Work out the finished part from the listing and answer in its coordinate system (mm). Face numbers are marked on the shaded views. A direction names the side the tool comes from. Coordinates: 2 decimals unless noted, no trailing zeros. Write each question's results on one line, items separated by ' | '. Start each with the question number.
Item 1: Section C-C, the plane y = 28.5 is taken. Count the separate pieces of the cut face and the enclosed holes in it, plus the area to 3 significant figures.
Item 2: Each of these flat-tipped pins is pushed along its axis until it touches: pin 1 Ø2.5 at (x, y) = (-1, 43.5) entering from +Z; pin 2 Ø3.5 at (x, z) = (65.5, -3.5) entering from -Y; pin 3 Ø13.5 at (x, y) = (-17, 24) entering from -Z. Where does it stop, or does it pass through?
Item 3: Consider probe 1 along Z at (x, y) = (-5.5, 29); probe 2 along Z at (x, y) = (-44, 42); probe 3 along X at (y, z) = (14, -38) (3 decimals). Determine where each line is inside the solid, lowest interval first. Write a range as [from, to].
Item 4: A tool of negligible diameter and unlimited length cuts with its end or side. For the marked faces 4, 5 and 6, from which of +Z, -Z, +X, -X, +Y, -Y can it reach the whole face along a straight path? Write none if from no direction.
Item 5: For a pull along Z with two mould halves and no side action, classify the marked faces 1, 2 and 3 as +Z half, -Z half, draft (parallel to the pull), parting line (faces both ways), or undercut.
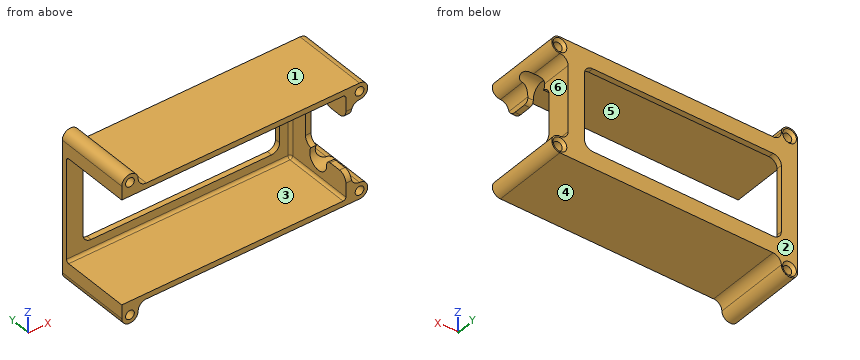
from build123d import *

# Parameters (mm, degrees)
SKETCH1_W           = 133.35
SKETCH1_H           = 66.675
SKETCH1_W_2         = 127
SKETCH1_H_2         = 60.325
BOSS_EXTRUDE1_DEPTH = 41.275
SKETCH2_W           = 31.75
SKETCH2_H           = 60.325
CUT_EXTRUDE1_DEPTH  = 134.35
SKETCH3_W           = 133.35
SKETCH3_H           = 66.675
SKETCH3_W_2         = 114.3
SKETCH3_H_2         = 47.625
BOSS_EXTRUDE2_DEPTH = 3.175
BOSS_EXTRUDE3_DEPTH = 44.45
SKETCH6_R           = 2.54
BOSS_EXTRUDE4_DEPTH = 44.45
CUT_EXTRUDE2_DEPTH  = 4.175
FILLET1_R           = 1.5875
FILLET2_R           = 4.7625
SKETCH9_R           = 6.35
CUT_EXTRUDE4_DEPTH  = 13.7
FILLET3_R           = 2.54


with BuildPart() as part:
    # Sketch1 → Boss-Extrude1 (new body)
    with BuildSketch(Plane(origin=(0, 0, 0), x_dir=(1, 0, 0), z_dir=(0, 1, 0))):
        Rectangle(SKETCH1_W, SKETCH1_H)
        Rectangle(SKETCH1_W_2, SKETCH1_H_2, mode=Mode.SUBTRACT)
    extrude(amount=BOSS_EXTRUDE1_DEPTH)

    # Sketch2 → Cut-Extrude1 (cut, through all)
    with BuildSketch(Plane.ZY.offset(66.675)):
        Rectangle(SKETCH2_W, SKETCH2_H)
    extrude(amount=-CUT_EXTRUDE1_DEPTH, mode=Mode.SUBTRACT)

    # Sketch3 → Boss-Extrude2 (add)
    with BuildSketch(Plane(origin=(0, 41.275, 0), x_dir=(1, 0, 0), z_dir=(0, 1, 0))):
        Rectangle(SKETCH3_W, SKETCH3_H)
        Rectangle(SKETCH3_W_2, SKETCH3_H_2, mode=Mode.SUBTRACT)
    extrude(amount=BOSS_EXTRUDE2_DEPTH)

    # Sketch4 → Boss-Extrude3 (add)
    with BuildSketch(Plane(origin=(0, 44.45, 0), x_dir=(1, 0, 0), z_dir=(0, 1, 0))):
        with BuildLine():
            Line((71.4375, 33.3375), (66.675, 33.3375))
            Line((66.675, 33.3375), (66.675, 19.05))
            ThreePointArc((66.675, 19.05), (68.069903955, 22.417596045), (71.4375, 23.8125))
            ThreePointArc((71.4375, 23.8125), (76.2, 28.575), (71.4375, 33.3375))
        make_face()
    boss_extrude3 = extrude(amount=-BOSS_EXTRUDE3_DEPTH)

    # Sketch5 → Cut-Revolve1 (revolve, cut)
    with BuildSketch(Plane.YZ.offset(71.4375)):
        Polygon((0, -31.115), (42.8625, -31.115), (44.45, -32.569675739), (44.45, -28.575), (0, -28.575), align=None)
    cut_revolve1 = revolve(axis=Axis((71.4375, 44.45, -28.575), (0, -1, 0)), mode=Mode.SUBTRACT)

    # Sketch6 → Boss-Extrude4 (add)
    with BuildSketch(Plane(origin=(0, 44.45, 0), x_dir=(1, 0, 0), z_dir=(0, 1, 0))):
        with BuildLine():
            Line((-66.675, 38.1), (-66.675, 33.3375))
            Line((-66.675, 33.3375), (-52.3875, 33.3375))
            ThreePointArc((-52.3875, 33.3375), (-55.755096045, 34.732403955), (-57.15, 38.1))
            ThreePointArc((-57.15, 38.1), (-61.9125, 42.8625), (-66.675, 38.1))
        make_face()
        with Locations((-61.9125, 38.1)):
            Circle(SKETCH6_R, mode=Mode.SUBTRACT)
    boss_extrude4 = extrude(amount=-BOSS_EXTRUDE4_DEPTH)

    # Sketch7 → Cut-Revolve2 (revolve, cut)
    with BuildSketch(Plane(origin=(-61.9125, 0, 0), x_dir=(0, 1, 0), z_dir=(-1, 0, 0))):
        Polygon((42.8625, 40.64), (44.45, 42.094675739), (44.45, 38.1), (42.8625, 38.1), align=None)
    cut_revolve2 = revolve(axis=Axis((-61.9125, 42.8625, -38.1), (0, -1, 0)), mode=Mode.SUBTRACT)

    # Mirror1: Boss-Extrude3, Cut-Revolve1, Boss-Extrude4, Cut-Revolve2 across plane
    add(boss_extrude3.mirror(Plane.XY))
    add(cut_revolve1.mirror(Plane.XY), mode=Mode.SUBTRACT)
    add(boss_extrude4.mirror(Plane.XY))
    add(cut_revolve2.mirror(Plane.XY), mode=Mode.SUBTRACT)

    # Sketch8 → Cut-Extrude2 (cut, through all)
    with BuildSketch(Plane(origin=(-63.5, 0, 0), x_dir=(0, 0, -1), z_dir=(1, 0, 0))):
        Polygon((-15.875, 0), (-15.875, 30.1625), (15.875, 30.1625), (15.875, 0), (30.1625, 0), (30.1625, 41.275), (-30.1625, 41.275), (-30.1625, 0), align=None)
    extrude(amount=-CUT_EXTRUDE2_DEPTH, mode=Mode.SUBTRACT)

    # Fillet1
    fillet1_edges = [part.edges().sort_by_distance(p)[0] for p in [
        (63.5, 20.6375, 30.1625),
        (63.5, 20.6375, -30.1625),
        (63.5, 41.275, 0),
        (-1.5875, 41.275, -30.1625),
        (-1.5875, 41.275, 30.1625),
    ]]
    fillet(fillet1_edges, radius=FILLET1_R)

    # Fillet2
    fillet2_edges = [part.edges().sort_by_distance(p)[0] for p in [
        (65.0875, 0, 15.875),
        (65.0875, 30.1625, 15.875),
        (65.0875, 0, -15.875),
        (65.0875, 30.1625, -15.875),
        (-57.15, 42.8625, 23.8125),
        (57.15, 42.8625, 23.8125),
        (57.15, 42.8625, -23.8125),
        (-57.15, 42.8625, -23.8125),
    ]]
    fillet(fillet2_edges, radius=FILLET2_R)

    # Sketch9 → Cut-Extrude4 (cut, through all)
    with BuildSketch(Plane.ZY.offset(-63.5)):
        with Locations((19.05, 20.6375)):
            Circle(SKETCH9_R)
        with Locations((-19.05, 20.6375)):
            Circle(SKETCH9_R)
    extrude(amount=-CUT_EXTRUDE4_DEPTH, mode=Mode.SUBTRACT)

    # Fillet3
    fillet3_edges = [part.edges().sort_by_distance(p)[0] for p in [
        (65.0875, 15.138238686, 15.875),
        (65.0875, 15.138238686, -15.875),
    ]]
    fillet(fillet3_edges, radius=FILLET3_R)


solid = part.part
Answer key:
1) separate pieces: 2 | enclosed holes: 4 | area: 1,210 mm^2
2) pin 1: stops at z = 33.34 | pin 2: stops at y = 30.16 | pin 3: stops at z = -33.34
3) probe 1: z = [-33.34, -30.16], [30.16, 33.34] | probe 2: z = [-33.34, -23.81], [23.81, 33.34] | probe 3: x = [-66.675, -64.451], [-59.374, -57.149]
4) face 4: -Z, +X, +Y, -Y | face 5: -X, -Y | face 6: +X, +Y, -Y
5) face 1: +Z half | face 2: draft | face 3: undercut
